Here's the drawing with two shaded views (mm, measured from the low corner). I have some questions. A direction names the side the tool comes from. Coordinates: 2 decimals unless noted, no trailing zeros. Write each loop counter-clockwise with the first axis right and the second up, starting at its lowest first coordinate (ties: lowest second). Pieces come first, ordered by that corner, then holes. Notation, with made-up numbers: (18, 59) -> (63, 59) arc R21 cw to (63, 68) -> close; hole circle Ø6 at (-31.5, -32). An arc over 180 degrees is marked (long way). Put each result on its own line as item: value.
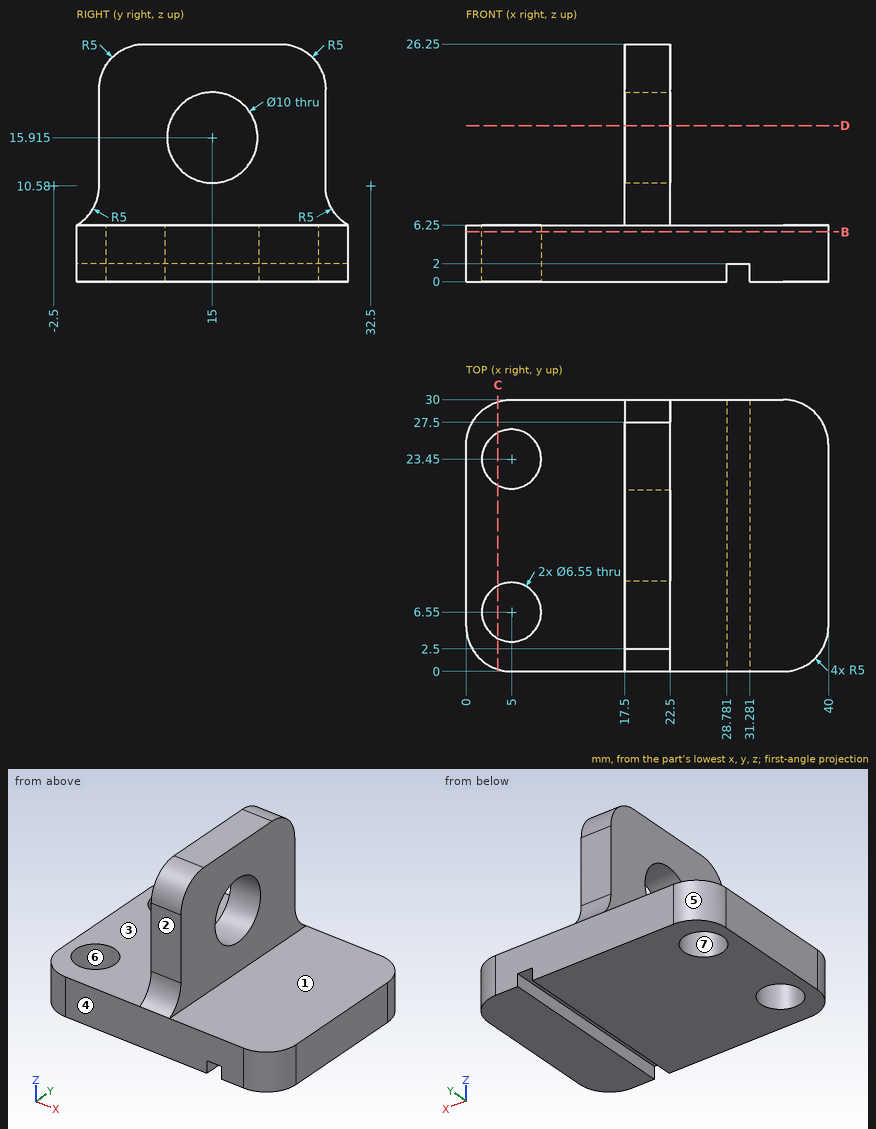
Item 1: If we mould it in two halves opening along X, with no side actions, what happens to the marked faces 4, 5, 6 and 7? For each: released by +X, released by -X, zero draft, split by the parting line, or undercut.
Output:
face 4: zero draft
face 5: released by -X
face 6: undercut
face 7: undercut
Item 2: Which directions (+Z, -Z, +X, -X, +Y, -Y) give clear straight access to the entire face, cutting with the end or side of a thin tool? Please do the marked faces 1, 2 and 3.
Output:
face 1: +Z, +X, +Y, -Y
face 2: +Z, +X, -X, -Y
face 3: +Z, -X, +Y, -Y
Item 3: Please list where these lines run through material, in increasing order: line 1 along Y through (x, z) = (5, 2.5) (1 decimal); line 2 along X through (y, z) = (14, 1.75); line 3 along Y through (x, z) = (7.5, 2) (1 decimal). Write a range as from..to.
Output:
line 1: y = 0..3.3, 9.8..20.2, 26.7..30
line 2: x = 0..28.78, 31.28..40
line 3: y = 0..4.4, 8.7..21.3, 25.6..30
Item 4: Imagine slicing it at B-B on z = 5.5. State how many separate pieces and enclosed holes the cut face has, then the cut area to 3 significant figures.
Output:
separate pieces: 1
enclosed holes: 2
area: 1,110 mm²
Item 5: Imagine slicing it at C-C on x = 3.5. Write out the boundary of the cut face in (y, z), then the cut area to 3 significant figures.
Output:
outline: (0.23, 0) -> (3.64, 0) -> (3.64, 6.25) -> (0.23, 6.25) -> close; (9.46, 0) -> (20.54, 0) -> (20.54, 6.25) -> (9.46, 6.25) -> close; (26.36, 0) -> (29.77, 0) -> (29.77, 6.25) -> (26.36, 6.25) -> close
area: 112 mm²
Item 6: Imagine slicing it at D-D on z = 17.25. Write out the boundary of the cut face in (x, y).
Output:
outline: (17.5, 2.5) -> (22.5, 2.5) -> (22.5, 10.18) -> (17.5, 10.18) -> close; (17.5, 19.82) -> (22.5, 19.82) -> (22.5, 27.5) -> (17.5, 27.5) -> close
Item 7: For P1, Ø10, axis at y = 8, z = 20, coming from the -X side; P2, Ø5, axis at x = 9.5, y = 21, coming from the +Z side; P3, Ø0.8, axis at x = 30.5, y = 20, coming from the -Z side; P4, Ø6, axis at y = 15, z = 15.92, coming from the -X side, each with a flat end and sliding along its axis, tell me the tip position at first contact or that it passes through.
Output:
P1: stops at x = 17.5
P2: stops at z = 6.25
P3: stops at z = 2
P4: passes through
